```python
from build123d import *

# Parameters (mm, degrees)
BOSS_EXTRUDE1_DEPTH = 5.8
CUT_EXTRUDE1_DEPTH  = 83.286876232
FILLET1_R           = 1


with BuildPart() as part:
    # Sketch1 → Boss-Extrude1 (new body)
    with BuildSketch(Plane.XY):
        Polygon((0, 0), (90, 0), (90, 6), (80.7, 6), (80.7, 15), (72.8, 15), (72.8, 6), (17.2, 6), (17.2, 15), (9.3, 15), (9.3, 6), (0, 6), align=None)
    extrude(amount=BOSS_EXTRUDE1_DEPTH)

    # Sketch2 → Cut-Extrude1 (cut, through all)
    with BuildSketch(Plane(origin=(80.7, 0, 0), x_dir=(0, 0, -1), z_dir=(1, 0, 0))):
        Polygon((-5.8, 15), (-5.8, 6), (-4.8, 15), align=None)
    extrude(amount=-CUT_EXTRUDE1_DEPTH, mode=Mode.SUBTRACT)

    # Fillet1
    fillet1_edges = [part.edges().sort_by_distance(p)[0] for p in [
        (0, 6, 2.9),
        (90, 6, 2.9),
        (90, 0, 2.9),
        (0, 0, 2.9),
        (9.3, 15, 2.4),
        (17.2, 15, 2.4),
        (72.8, 15, 2.4),
        (80.7, 15, 2.4),
    ]]
    fillet(fillet1_edges, radius=FILLET1_R)


solid = part.part
```
Input: part model. Units: mm. Frame: model coordinates. A direction names the side the tool comes from. Give positions to 0.01 mm unless a question says otherwise; leave off trailing zeros. Write each loop counter-clockwise with the first axis right and the second up, starting at its lowest first coordinate (ties: lowest second). Pieces come first, ordered by that corner, then holes. Notation, with made-up numbers: (-39.5, 50.5) - (15.5, 50.5) arc R23 ccw to (15.5, 70.5) - close; hole circle Ø2 at (12.25, -6). An arc over 180 degrees is marked (long way). Write item = value, one per line. Start each with the question number.
1) Pin query (flat end, axial travel): pin 1 (1 mm diameter, centred on x = 16, y = 8.5, fed in from +Z); pin 2 (3 mm diameter, centred on y = 11, z = 3.5, fed in from -X); pin 3 (3 mm diameter, centred on y = 7, z = 1.5, fed in from +X); pin 4 (6 mm diameter, centred on x = 41, y = 8.5, fed in from +Z). Return the tip coordinate at first contact, or that it passes through.
2) Material intervals for L1, parallel to X at y = 12.25, z = 0.5; L2, parallel to Y at x = 65, z = 4.2; L3, parallel to X at y = 5.5, z = 3.9, sorted ascending. Write a range as [from, to].
3) Draft query along X for faces 5 (the face through (17.2, 10, 3)), 6 (the face through (76.805, 10.437, 5.307)), 7 (the face through (90, 3, 3)). Return one class per face: pulls with the +X half, pulls with the -X half, needs draft (parallel to the pull), parting line crosses it, or undercut.
4) Cut plane A-A (y = 8.5). Return loops of the section in (x, z), and give its area (3 significant figures).
5) Reachability of faces 1 (the face through (77, 15, 2)), 2 (the face through (72.8, 10, 3)), 3 (the face through (85, 6, 3)), 4 (the face through (5, 6, 3)) from +Z, -Z, +X, -X, +Y, -Y: full face, straight path, thin tool, end or side. Return the list, or none.
6) Cut plane C-C (x = 76). Return loops of the section in (y, z), and give its area (3 significant figures).
7) Cut plane D-D (x = 20). Return loops of the section in (y, z), and give its area (3 significant figures).
8) Cut plane B-B (z = 3). Return loops of the section in (x, y), and give its area (3 significant figures).
Answers follow:
q1.pin_1 = 5.58
q1.pin_2 = 9.3
q1.pin_3 = 89.87
q1.pin_4 = 5.8
q2.L1 = [9.3, 17.2], [72.8, 80.7]
q2.L2 = [0, 6]
q2.L3 = [0.13, 89.87]
q3.face_5 = undercut
q3.face_6 = needs draft
q3.face_7 = pulls with the +X half
q4.outline = (9.3, 0) - (17.2, 0) - (17.2, 5.52) - (9.3, 5.52) - close; (72.8, 0) - (80.7, 0) - (80.7, 5.52) - (72.8, 5.52) - close
q4.area = 87.3 mm^2
q5.face_1 = +Z, -Z, +X, -X, +Y
q5.face_2 = +Z, -Z, +Y
q5.face_3 = +Z, -Z, +X, +Y
q5.face_4 = +Z, -Z, -X, +Y
q6.outline = (0, 0) - (15, 0) - (15, 4.8) - (6, 5.8) - (0, 5.8) - close
q6.area = 82.5 mm^2
q7.outline = (0, 0) - (6, 0) - (6, 5.8) - (0, 5.8) - close
q7.area = 34.8 mm^2
q8.outline = (0, 1) arc R1 ccw to (1, 0) - (89, 0) arc R1 ccw to (90, 1) - (90, 5) arc R1 ccw to (89, 6) - (80.7, 6) - (80.7, 14) arc R1 ccw to (79.7, 15) - (73.8, 15) arc R1 ccw to (72.8, 14) - (72.8, 6) - (17.2, 6) - (17.2, 14) arc R1 ccw to (16.2, 15) - (10.3, 15) arc R1 ccw to (9.3, 14) - (9.3, 6) - (1, 6) arc R1 ccw to (0, 5) - close
q8.area = 680 mm^2
